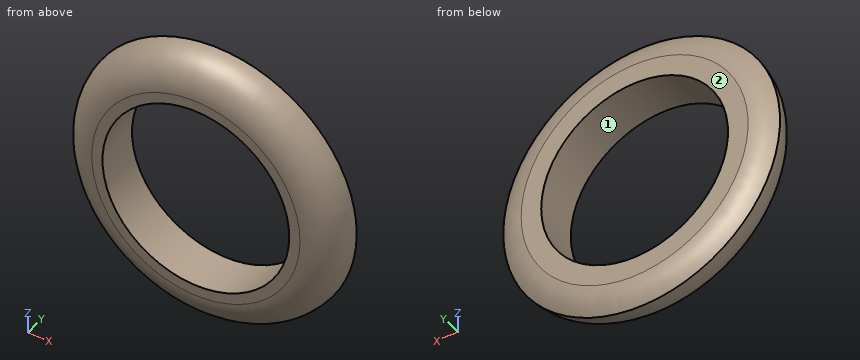
```python
from build123d import *

# Parameters (mm, degrees)
F2_R     = 20.5358515241
F2_R_2   = 13.8603934158
F0_DEPTH = 6.6770780832
F3_R     = 5.08


# Not quite as in the source:
# - a fillet or chamfer that OpenCascade refuses, or shapes differently, is made with other operations: its cross-section is extruded or revolved along the edge and cut away or added


with BuildPart() as f0:
    # F2 (on Front) → F0 (new body)
    with BuildSketch(Plane.XZ):
        Circle(F2_R)
        Circle(F2_R_2, mode=Mode.SUBTRACT)
    extrude(amount=F0_DEPTH)

    # F3
    f3_edges = [f0.edges().sort_by_distance(p)[0] for p in [
        (-20.535852, -6.677078, 0),
    ]]
    fillet(f3_edges, radius=F3_R)

    # F1: fillet of radius 5.08 on 1 edges, made by hand

    # F1_s1 → F1_t2 (revolve, cut)
    with BuildSketch(Plane.XY):
        with BuildLine():
            ThreePointArc((20.5358515241, -1.5970780832), (18.8518854725, -0.4163295926), (16.8377905564, 0))
            Line((16.8377905564, 0), (20.5358515241, 0))
            Line((20.5358515241, 0), (20.5358515241, -1.5970780832))
        make_face()
    revolve(axis=Axis((0, 0, 0), (0, -1, 0)), mode=Mode.SUBTRACT)


solid = f0.part
```
Source: CAD feature listing. Evaluate the final solid. Frame: model axes, mm. Face numbers are marked on the shaded views. Coordinates: 2 decimals unless noted, no trailing zeros. Loops run counter-clockwise (first coordinate to the right, second up) from the corner with the lowest first, then second, coordinate; pieces in that order, holes last. Notation, with made-up numbers: (51, -10) -> (101, -10) arc R21 ccw to (101, 20) -> close; hole circle Ø2 at (27, 34). An arc over 180 degrees is marked (long way). One line per item, written item: value. Start each with the question number.
Q1. Section query A-A, the plane x = 0. Return the cut outline in (y, z).
Q2. Section query C-C, the plane y = -0.5. Return the cut outline in (x, z), and give its area (3 significant figures).
Q3. Section query D-D, the plane y = -6. Return the cut outline in (x, z), and give its area (3 significant figures).
Q4. Section query B-B, the plane z = 0. Return the cut outline in (x, y).
Q5. Line query: line 1 along Z through (x, y) = (-9, -5.25); line 2 along X through (y, z) = (-2.25, -5); line 3 along Z through (x, y) = (0, -4.5). Output: solid intervals per line, ascending.
Q6. Mould query, pull axis X, two halves, no side actions, for the marked faces 1 and 2. Classes: pulls with the +X half, pulls with the -X half, needs draft (parallel to the pull), parting line crosses it, or undercut.
Q7. Contact query for a flat-ended pin moving along its axis: P1, Ø10, axis at x = 0.5, z = -10, coming from the +Y side. Output: stop coordinate, or through.
Results:
1. outline: (-6.68, -15.46) arc R5.08 ccw to (-1.6, -20.54) arc R5.08 ccw to (0, -16.84) -> (0, -13.86) -> (-6.68, -13.86) -> close; (-6.68, 13.86) -> (0, 13.86) -> (0, 16.84) arc R5.08 ccw to (-1.6, 20.54) arc R5.08 ccw to (-6.68, 15.46) -> close
2. outline: circle Ø38.07 at (0, 0); hole circle Ø27.72 at (0, 0)
2. area: 535 mm^2
3. outline: circle Ø35.98 at (0, 0); hole circle Ø27.72 at (0, 0)
3. area: 413 mm^2
4. outline: (-20.54, -1.6) arc R5.08 ccw to (-15.46, -6.68) -> (-13.86, -6.68) -> (-13.86, 0) -> (-16.84, 0) arc R5.08 ccw to start; (13.86, -6.68) -> (15.46, -6.68) arc R5.08 ccw to (20.54, -1.6) arc R5.08 ccw to (16.84, 0) -> (13.86, 0) -> close
5. line 1: -16.72 to -10.54, 10.54 to 16.72
5. line 2: -19.87 to -12.93, 12.93 to 19.87
5. line 3: -19.62 to -13.86, 13.86 to 19.62
6. face 1: undercut
6. face 2: needs draft
7. P1: y = 0
